```python
from build123d import *

# Parameters (mm, degrees)
F0_W     = 290
F0_H     = 225
F1_DEPTH = 2
F2_W     = 40
F2_H     = 225
F2_H_2   = 40
F3_DEPTH = 125
F4_W     = 185
F4_H     = 140
F5_DEPTH = 165
F6_W     = 185
F6_H     = 60
F7_DEPTH = 55
F8_W     = 25.804932
F8_H     = 140
F9_DEPTH = 165


with BuildPart() as f1:
    # F0 (on Top) → F1 (new body)
    with BuildSketch(Plane.XY):
        with Locations((31.78409, 48.083462)):
            Rectangle(F0_W, F0_H)
    extrude(amount=F1_DEPTH)

    # F2 (on face) → F3 (join)
    with BuildSketch(Plane.XY.offset(2)):
        with Locations((-28.21591, 48.083462)):
            Rectangle(F2_W, F2_H)
        with Locations((-28.21591, -84.416538)):
            Rectangle(F2_W, F2_H_2)
    extrude(amount=F3_DEPTH)

    # F4 (on face) → F5 (join)
    with BuildSketch(Plane.XY.offset(2)):
        with Locations((84.28409, 90.583462)):
            Rectangle(F4_W, F4_H)
    extrude(amount=F5_DEPTH)

    # F6 (on face) → F7 (join)
    with BuildSketch(Plane.XY.offset(2)):
        with Locations((84.28409, -9.416538)):
            Rectangle(F6_W, F6_H)
    extrude(amount=F7_DEPTH)

    # F8 (on face) → F9 (cut)
    with BuildSketch(Plane.XY.offset(167)):
        with Locations((163.881624, 90.583462)):
            Rectangle(F8_W, F8_H)
    extrude(amount=-F9_DEPTH, mode=Mode.SUBTRACT)


solid = f1.part
```
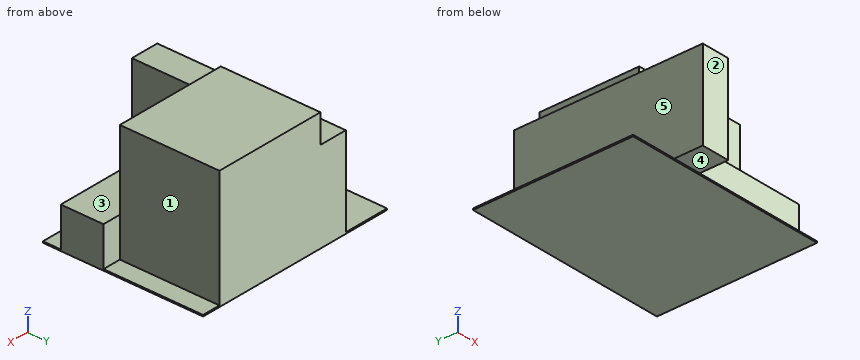
Geometry check sheet. Reference: the model listing, model coordinates, mm. Face numbers are marked on the shaded views. A direction names the side the tool comes from. Coordinates: 2 decimals unless noted, no trailing zeros. Loops run counter-clockwise (first coordinate to the right, second up) from the corner with the lowest first, then second, coordinate; pieces in that order, holes last. Notation, with made-up numbers: (77.25, 53.25) -> (130.25, 53.25) arc R26 ccw to (130.25, 68.25) -> close; hole circle Ø10 at (0.5, 86). An arc over 180 degrees is marked (long way). Put each result on its own line as item: value.
1) Cross-section at A-A on y = 7. Record the boundary of the cut face in (x, z), plus the area to 3 significant figures.
Result set:
outline: (-113.22, 0) -> (176.78, 0) -> (176.78, 57) -> (-8.22, 57) -> (-8.22, 127) -> (-48.22, 127) -> (-48.22, 2) -> (-113.22, 2) -> close
area: 15,800 mm^2
2) Cross-section at B-B on z = 67. Record the boundary of the cut face in (x, y), plus the area to 3 significant figures.
Result set:
outline: (-48.22, -104.42) -> (-8.22, -104.42) -> (-8.22, 20.58) -> (150.98, 20.58) -> (150.98, 160.58) -> (-48.22, 160.58) -> close
area: 32,900 mm^2
3) Thickness scan on line 1 (X direction, y = -80.5, z = 120); line 2 (Y direction, x = 79.5, z = 121); line 3 (Y direction, x = 42.5, z = 49). Record the ranges inside material, lowest first.
Result set:
line 1: x = -48.22 to -8.22
line 2: y = 20.58 to 160.58
line 3: y = -39.42 to 160.58
4) Cross-section at D-D on y = 42. Record the boundary of the cut face in (x, z).
Result set:
outline: (-113.22, 0) -> (176.78, 0) -> (176.78, 2) -> (150.98, 2) -> (150.98, 167) -> (-8.22, 167) -> (-8.22, 127) -> (-48.22, 127) -> (-48.22, 2) -> (-113.22, 2) -> close
5) Cross-section at C-C on x = 49. Record the boundary of the cut face in (y, z).
Result set:
outline: (-64.42, 0) -> (160.58, 0) -> (160.58, 167) -> (20.58, 167) -> (20.58, 57) -> (-39.42, 57) -> (-39.42, 2) -> (-64.42, 2) -> close
6) Tool access check on the marked faces 1, 2, 3, 4 and 5. Record the directions out of +Z, -Z, +X, -X, +Y, -Y that give a thin tool (end or side, any length) a straight path to the whole face; none if there is none.
Result set:
face 1: +Z, +X, +Y
face 2: +Z, -Z, +X, -X, -Y
face 3: +Z, +X, -Y
face 4: -Z, +X, -X, -Y
face 5: +Z, -X, +Y, -Y
7) Gauge pin test, flat ends, axial feed: pin 1 Ø12 at (y, z) = (81, 139.5) entering from -X; pin 2 Ø7.5 at (x, z) = (164, 36) entering from +Y; pin 3 Ø12 at (y, z) = (98.5, 129) entering from -X. Record the tip position at first contact, or that the pin passes through.
Result set:
pin 1: stops at x = -8.22
pin 2: stops at y = 20.58
pin 3: stops at x = -48.22
